from build123d import *

# Parameters (mm, degrees)
ESBO_O2_W                = 8
ESBO_O2_H                = 28
RESSALTO_EXTRUS_O1_DEPTH = 2.5
ESBO_O3_W                = 3
ESBO_O3_H                = 0.6
CORTE_EXTRUS_O1_DEPTH    = 25
ESBO_O4_W                = 2.5
ESBO_O4_H                = 2
RESSALTO_EXTRUS_O2_DEPTH = 20


with BuildPart() as part:
    # Esboço2 → Ressalto-extrusão1 (new body)
    with BuildSketch(Plane.XY):
        Rectangle(ESBO_O2_W, ESBO_O2_H)
    extrude(amount=RESSALTO_EXTRUS_O1_DEPTH)

    # Esboço3 → Corte-extrusão1 (cut)
    with BuildSketch(Plane.XZ.offset(14)):
        with Locations((0, 1.25)):
            Rectangle(ESBO_O3_W, ESBO_O3_H)
    extrude(amount=-CORTE_EXTRUS_O1_DEPTH, mode=Mode.SUBTRACT)

    # Esboço4 → Ressalto-extrusão2 (add)
    with BuildSketch(Plane(origin=(4, 0, 0), x_dir=(0, 0, -1), z_dir=(1, 0, 0))):
        with Locations((-1.25, 13)):
            Rectangle(ESBO_O4_W, ESBO_O4_H)
        with Locations((-1.25, 9)):
            Rectangle(ESBO_O4_W, ESBO_O4_H)
    extrude(amount=RESSALTO_EXTRUS_O2_DEPTH)


solid = part.part
Part model, mm, in its own coordinate system. A direction names the side the tool comes from. Coordinates: 2 decimals unless noted, no trailing zeros. Loops run counter-clockwise (first coordinate to the right, second up) from the corner with the lowest first, then second, coordinate; pieces in that order, holes last. Notation, with made-up numbers: (69.25, -20) -> (99.25, -20) arc R29 cw to (99.25, 9) -> close; hole circle Ø9 at (11, -29). An arc over 180 degrees is marked (long way). Use a Markdown table: item, result. Add a question column.
Item 1: Pull direction X, two halves, no side cores. Call faces 4 (the flat face through (24, 13, 1)), 5 (the flat face through (3.6, 2.9, 2.5)), 6 (the flat face through (0, -2, 0.95)): +X half, -X half, draft (parallel to the pull), parting line (faces both ways), or undercut.
Item 2: Band-saw the part on D-D on x = 0.5. Write the cut outline in (y, z).
Item 3: Band-saw the part on A-A on x = 8.25. Write the cut outline in (y, z).
Item 4: Flat gauge pins, fed straight in: P1, Ø0.7, axis at y = -3, z = 1.5, coming from the +X side; P2, Ø1.2, axis at x = 13, z = 1, coming from the -Y side. Where does each tip first touch, or does it go through?
Item 5: Which spindle directions (+Z, -Z, +X, -X, +Y, -Y) get a long thin tool onto all of the face, cutting with end or side? Do faces 1 (the flat face through (14, 10, 1)), 2 (the flat face through (4, -3, 1)), 3 (the flat face through (0, -2, 1.55)). Say none if no direction does.
Item 6: Band-saw the part on B-B on y = 2.75. Write the cut outline in (x, z), plus the area to 3 significant figures.
Item 7: Band-saw the part on C-C on z = 0.55. Write the cut outline in (x, y).
Item 8: Probe probe 1 along Y at (x, z) = (6, 2.3); probe 2 along X at (y, z) = (-1.5, 1); probe 3 along Z at (x, y) = (0, 8.75). List the from-to ranges inside material, lowest first.
Geometry says:
| question | item | result |
|---|---|---|
| 1 | face 4 | +X half |
| 1 | face 5 | draft |
| 1 | face 6 | undercut |
| 2 | outline | (-14, 0) -> (14, 0) -> (14, 2.5) -> (-14, 2.5) -> (-14, 1.55) -> (11, 1.55) -> (11, 0.95) -> (-14, 0.95) -> close |
| 3 | outline | (8, 0) -> (10, 0) -> (10, 2.5) -> (8, 2.5) -> close; (12, 0) -> (14, 0) -> (14, 2.5) -> (12, 2.5) -> close |
| 4 | P1 | x = 4 |
| 4 | P2 | y = 8 |
| 5 | face 1 | +Z, -Z, +X |
| 5 | face 2 | +Z, -Z, +X, -Y |
| 5 | face 3 | -Y |
| 6 | outline | (-4, 0) -> (4, 0) -> (4, 2.5) -> (-4, 2.5) -> close; hole (-1.5, 0.95) -> (1.5, 0.95) -> (1.5, 1.55) -> (-1.5, 1.55) -> close |
| 6 | area | 18.2 mm² |
| 7 | outline | (-4, -14) -> (4, -14) -> (4, 8) -> (24, 8) -> (24, 10) -> (4, 10) -> (4, 12) -> (24, 12) -> (24, 14) -> (-4, 14) -> close |
| 8 | probe 1 | 8 to 10, 12 to 14 |
| 8 | probe 2 | -4 to -1.5, 1.5 to 4 |
| 8 | probe 3 | 0 to 0.95, 1.55 to 2.5 |
